Geometry check sheet. Reference: the model listing, model coordinates, mm. A direction names the side the tool comes from. Give positions to 0.01 mm unless a question says otherwise; leave off trailing zeros. Loops run counter-clockwise (first coordinate to the right, second up) from the corner with the lowest first, then second, coordinate; pieces in that order, holes last.
1. Go/stop test with flat-tipped pins: pin 1 Ø10 at (x, z) = (20.5, -31.5) entering from +Y; pin 2 Ø1 at (x, y) = (17.5, 18) entering from +Z; pin 3 Ø8 at (x, y) = (19.5, 29.5) entering from -Z. Record where each tip stops, or that it passes through.
2. Cross-section at B-B, the plane x = 14.5. Record the cut outline in (y, z), plus the area to 3 significant figures.
3. Tool access check on faces 1 (the flat face through (-10, -1, -69.469)), 2 (the cylindrical face through (12.522, -6.108, -40.547)), 3 (the cylindrical face through (12.5, 47.6, 30.2)), 4 (the cylindrical face through (12.52, -25.54, -20.99)). Record the directions out of +Z, -Z, +X, -X, +Y, -Y that give a thin tool (end or side, any length) a straight path to the whole face; none if there is none.
4. Cross-section at A-A, the plane z = 0. Record the cut outline in (x, y).
5. Material ranges on L1, parallel to X at y = 63, z = -12; L2, parallel to Z at x = 19, y = -6; L3, parallel to Y at x = 7.5, z = -36, recorded low to high.
6. Release check for a two-part mould opening along Z. For faces 5 (the flat face through (12.522, -29.66, -26.686)), 6 (the flat face through (12.522, -11.767, -44.714)), 7 (the flat face through (25.4, 12, -3)) record: +Z half, -Z half, draft (parallel to the pull), parting line (faces both ways), or undercut.
7. Cross-section at C-C, the plane y = 0. Record the cut outline in (x, z), plus the area to 3 significant figures.
from build123d import *

# Parameters (mm, degrees)
SKETCH1_W           = 138.938
SKETCH1_H           = 143.256
BOSS_EXTRUDE1_DEPTH = 20.32
BOSS_EXTRUDE2_DEPTH = 25.4


with BuildPart() as part:
    # Sketch1 → Boss-Extrude1 (new body)
    with BuildSketch(Plane(origin=(0, 0, 0), x_dir=(0, 0, -1), z_dir=(1, 0, 0))):
        Rectangle(SKETCH1_W, SKETCH1_H)
    extrude(amount=-BOSS_EXTRUDE1_DEPTH)

    # Sketch2 → Boss-Extrude2 (add)
    with BuildSketch(Plane(origin=(0, 0, 0), x_dir=(0, 0, -1), z_dir=(1, 0, 0))):
        with BuildLine():
            Line((47.080256121, -14.133743879), (42.27993705, -9.333424808))
            ThreePointArc((42.27993705, -9.333424808), (40.536989709, -6.056256364), (40.923806972, -2.364634654))
            ThreePointArc((40.923806972, -2.364634654), (-31.430896424, 46.416896424), (17.350634654, -25.937806972))
            ThreePointArc((17.350634654, -25.937806972), (21.042256364, -25.550989709), (24.319424808, -27.29393705))
            Line((24.319424808, -27.29393705), (29.119743879, -32.094256121))
            ThreePointArc((29.119743879, -32.094256121), (47.080256121, -32.094256121), (47.080256121, -14.133743879))
        make_face()
    extrude(amount=BOSS_EXTRUDE2_DEPTH)


solid = part.part
Result:
1. pin 1: stops at y = 50.67
1. pin 2: stops at z = 44.38
1. pin 3: stops at z = -43.19
2. outline: (-32.09, -29.12) arc R12.7 ccw to (-14.13, -47.08) - (-9.33, -42.28) arc R6.35 cw to (-2.36, -40.92) arc R44.45 ccw (long way) to (-25.94, -17.35) arc R6.35 cw to (-27.29, -24.32) - close
2. area: 6,720 mm2
3. face 1: -Z, +X, -X, +Y, -Y
3. face 2: -Z, +X
3. face 3: +X
3. face 4: +X, -Y
4. outline: (-20.32, -71.63) - (0, -71.63) - (0, -29.46) - (25.4, -29.46) - (25.4, 59.44) - (0, 59.44) - (0, 71.63) - (-20.32, 71.63) - close
5. L1: x = -20.32 to 0
5. L2: z = -40.53 to 39.18
5. L3: y = -35.64 to 41.06
6. face 5: undercut
6. face 6: -Z half
6. face 7: draft
7. outline: (-20.32, -69.47) - (0, -69.47) - (0, -41.85) - (25.4, -41.85) - (25.4, 41.85) - (0, 41.85) - (0, 69.47) - (-20.32, 69.47) - close
7. area: 4,950 mm2
